```python
from build123d import *

# Parameters (mm, degrees)
F0_W          = 5
F0_H          = 10
F0_R          = 1.55
F1_DEPTH      = 37
F2_W          = 15
F2_H          = 10
F3_DEPTH      = 4
F4_W          = 4.4
F4_H          = 10
F5_DEPTH      = 16.5
F6_R          = 2.5
F7_DEPTH      = 4.401
F7_DEPTH_BACK = 10.601
F8_W          = 3
F8_H          = 6
F9_DEPTH      = 10.001


# Not quite as in the source:
# - a feature names something its author has since deleted; it is built from what else it names


with BuildPart() as f1:
    # F0 (on Front) → F1 (new body)
    with BuildSketch(Plane.XZ):
        Rectangle(F0_W, F0_H)
        Circle(F0_R, mode=Mode.SUBTRACT)
    extrude(amount=F1_DEPTH)

    # F2 (on face) → F3 (join)
    with BuildSketch(Plane.XZ.offset(37)):
        Rectangle(F2_W, F2_H)
    extrude(amount=F3_DEPTH)

    # F4 (on face) → F5 (join)
    with BuildSketch(Plane.XZ.offset(41)):
        with Locations((-5.3, 0)):
            Rectangle(F4_W, F4_H)
        with Locations((5.3, 0)):
            Rectangle(F4_W, F4_H)
    extrude(amount=F5_DEPTH)

    # F6 (on face) → F7 (cut, two sides)
    with BuildSketch(Plane.YZ.offset(-3.1)) as f7_sk:
        with Locations((-52, 0)):
            Circle(F6_R)
    extrude(amount=-F7_DEPTH, mode=Mode.SUBTRACT)
    extrude(f7_sk.sketch, amount=F7_DEPTH_BACK, mode=Mode.SUBTRACT)

    # F8 (on face) → F9 (cut, through all)
    with BuildSketch(Plane(origin=(-2.5, 0, 0), x_dir=(0, -1, 0), z_dir=(-1, 0, 0))):
        with Locations((7.1113700978, 0)):
            Rectangle(F8_W, F8_H)
    extrude(amount=-F9_DEPTH, mode=Mode.SUBTRACT)


solid = f1.part
```
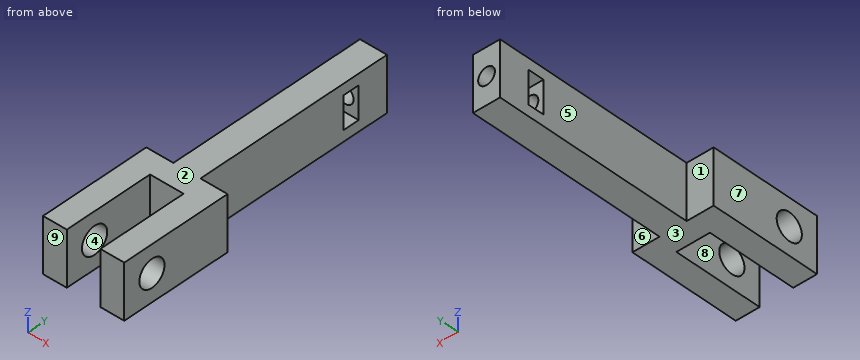
Here's how the part is built. I have some questions about the finished solid (model axes, mm). Face numbers are marked on the shaded views. A direction names the side the tool comes from. Coordinates: 2 decimals unless noted, no trailing zeros. Order: outer loops, then holes, each group sorted by start corner. A loop starts at its lowest first (then second) coordinate and runs counter-clockwise, first axis right, second up. Notation, with made-up numbers: M 44.25,-18 L 58.25,-18 A33 cw 58.25,20 Z; hole C 63,-10 d6. An arc over 180 degrees is marked long. Answer as a JSON object with one key per item and string values. Group by question number.
(1) If we mould it in two halves opening along Z, with no side actions, what happens to the marked faces 1, 2, 3 and 4? For each: released by +Z, released by -Z, zero draft, split by the parting line, or undercut.
(2) Suppose I cut it at A-A, the plane z = 0. State how many separate pieces and enclosed holes the cut face has, then the cut area to 3 significant figures.
(3) For pin 1 (5 mm diameter, centred on x = 0, z = 0.5, fed in from -Y); pin 2 (1 mm diameter, centred on y = -10.5, z = 2, fed in from -X); pin 3 (1.5 mm diameter, centred on x = 4, z = 0, fed in from +Y), each with a flat end and sliding along its axis, tell me the tip position at first contact or that it passes through.
(4) Which directions (+Z, -Z, +X, -X, +Y, -Y) give clear straight access to the entire face, cutting with the end or side of a thin tool? Please do the marked faces 5, 6, 7, 8 and 9.
(5) Suppose I cut it at D-D, the plane x = 0. Please give me the cut outline in (y, z), then the cut area to 3 significant figures.
(6) Suppose I cut it at B-B, the plane y = -50. Please give me the cut outline in (x, z), then the cut area to 3 significant figures.
(7) Suppose I cut it at C-C, the plane y = -7. Please give me the cut outline in (x, z).
(8) I need wall thicknesses on probe 1 along Z at (x, y) = (4.8, -52); probe 2 along X at (y, z) = (-45.5, 0); probe 3 along Z at (x, y) = (0, -4.5). Which ranges of each line are inside material? Lowest first, please.
Values found:
{
 "1": {"face 1": "zero draft", "face 2": "released by +Z", "face 3": "released by -Z", "face 4": "undercut"},
 "2": {"separate pieces": "5", "enclosed holes": "0", "area": "226 mm^2"},
 "3": {"pin 1": "stops at y = -41", "pin 2": "stops at x = -2.5", "pin 3": "stops at y = -37"},
 "4": {"face 5": "+Z, -Z, -X, +Y", "face 6": "+Z, -Z, +X, +Y", "face 7": "+Z, -Z, -X, +Y, -Y", "face 8": "+Z, -Z, -Y", "face 9": "+Z, -Z, +X, -X, -Y"},
 "5": {"outline": "M -41,-5 L 0,-5 L 0,-1.55 L -5.61,-1.55 L -5.61,-3 L -8.61,-3 L -8.61,-1.55 L -37,-1.55 L -37,1.55 L -8.61,1.55 L -8.61,3 L -5.61,3 L -5.61,1.55 L 0,1.55 L 0,5 L -41,5 Z", "area": "287 mm^2"},
 "6": {"outline": "M -7.5,-5 L -3.1,-5 L -3.1,-1.5 L -7.5,-1.5 Z; M -7.5,1.5 L -3.1,1.5 L -3.1,5 L -7.5,5 Z; M 3.1,-5 L 7.5,-5 L 7.5,-1.5 L 3.1,-1.5 Z; M 3.1,1.5 L 7.5,1.5 L 7.5,5 L 3.1,5 Z", "area": "61.6 mm^2"},
 "7": {"outline": "M -2.5,-5 L 2.5,-5 L 2.5,-3 L -2.5,-3 Z; M -2.5,3 L 2.5,3 L 2.5,5 L -2.5,5 Z"},
 "8": {"probe 1": "z = -5 to -2.5, 2.5 to 5", "probe 2": "x = -7.5 to -3.1, 3.1 to 7.5", "probe 3": "z = -5 to -1.55, 1.55 to 5"}
}
